```python
from build123d import *

# Parameters (mm, degrees)
SKETCH1_W           = 152.4
SKETCH1_H           = 457.2
SKETCH1_R           = 1.905
BOSS_EXTRUDE1_DEPTH = 4.7625
CUT_EXTRUDE1_REACH  = 411.779
SKETCH3_R           = 1.905
CUT_EXTRUDE4_REACH  = 411.779
SKETCH6_W           = 120.6373
SKETCH6_H           = 44.403792
SKETCH6_H_2         = 44.496208
SKETCH7_R           = 1.905
CUT_EXTRUDE5_DEPTH  = 410.778918528


with BuildPart() as part:
    # Sketch1 → Boss-Extrude1 (new body)
    with BuildSketch(Plane.XY):
        with Locations((-118.546343616, 131.913442623)):
            Rectangle(SKETCH1_W, SKETCH1_H)
        with Locations(Location((-61.396343616, 346.238642623, 0), (0, 0, 180))):
            Circle(SKETCH1_R, mode=Mode.SUBTRACT)
        with Locations(Location((-180.471543616, 346.238642623, 0), (0, 0, 180))):
            Circle(SKETCH1_R, mode=Mode.SUBTRACT)
        with Locations(Location((-180.471543616, -82.411757377, 0), (0, 0, 180))):
            Circle(SKETCH1_R, mode=Mode.SUBTRACT)
        with Locations(Location((-61.396343616, -82.411757377, 0), (0, 0, 180))):
            Circle(SKETCH1_R, mode=Mode.SUBTRACT)
    extrude(amount=BOSS_EXTRUDE1_DEPTH)

    # Sketch3 → Cut-Extrude1 (cut, up to next)
    with BuildSketch(Plane.XY.offset(4.7625), mode=Mode.PRIVATE) as cut_extrude1_sk1:
        with Locations((-156.633643616, 182.654534623)):
            Circle(SKETCH3_R)
    cut_extrude1_tool1 = extrude(cut_extrude1_sk1.sketch, amount=-CUT_EXTRUDE1_REACH, mode=Mode.PRIVATE) & part.part
    # Sketch3 → Cut-Extrude1 (cut, up to next)
    with BuildSketch(Plane.XY.offset(4.7625), mode=Mode.PRIVATE) as cut_extrude1_sk2:
        with Locations((-80.433643616, 182.654534623)):
            Circle(SKETCH3_R)
    cut_extrude1_tool2 = extrude(cut_extrude1_sk2.sketch, amount=-CUT_EXTRUDE1_REACH, mode=Mode.PRIVATE) & part.part
    # Sketch3 → Cut-Extrude1 (cut, up to next)
    with BuildSketch(Plane.XY.offset(4.7625), mode=Mode.PRIVATE) as cut_extrude1_sk3:
        with Locations((-156.633643616, 81.054534623)):
            Circle(SKETCH3_R)
    cut_extrude1_tool3 = extrude(cut_extrude1_sk3.sketch, amount=-CUT_EXTRUDE1_REACH, mode=Mode.PRIVATE) & part.part
    # Sketch3 → Cut-Extrude1 (cut, up to next)
    with BuildSketch(Plane.XY.offset(4.7625), mode=Mode.PRIVATE) as cut_extrude1_sk4:
        with Locations((-80.433643616, 81.054534623)):
            Circle(SKETCH3_R)
    cut_extrude1_tool4 = extrude(cut_extrude1_sk4.sketch, amount=-CUT_EXTRUDE1_REACH, mode=Mode.PRIVATE) & part.part
    add(cut_extrude1_tool1.solids().sort_by_distance((-156.633644, 182.654535, 4.7625))[0], mode=Mode.SUBTRACT)
    add(cut_extrude1_tool2.solids().sort_by_distance((-80.433644, 182.654535, 4.7625))[0], mode=Mode.SUBTRACT)
    add(cut_extrude1_tool3.solids().sort_by_distance((-156.633644, 81.054535, 4.7625))[0], mode=Mode.SUBTRACT)
    add(cut_extrude1_tool4.solids().sort_by_distance((-80.433644, 81.054535, 4.7625))[0], mode=Mode.SUBTRACT)

    # Sketch6 → Cut-Extrude4 (cut, up to next)
    with BuildSketch(Plane.XY.offset(4.7625), mode=Mode.PRIVATE) as cut_extrude4_sk1:
        with Locations((-118.539993616, 42.977638623)):
            Rectangle(SKETCH6_W, SKETCH6_H)
    cut_extrude4_tool1 = extrude(cut_extrude4_sk1.sketch, amount=-CUT_EXTRUDE4_REACH, mode=Mode.PRIVATE) & part.part
    # Sketch6 → Cut-Extrude4 (cut, up to next)
    with BuildSketch(Plane.XY.offset(4.7625), mode=Mode.PRIVATE) as cut_extrude4_sk2:
        with Locations((-118.539993616, 220.777638623)):
            Rectangle(SKETCH6_W, SKETCH6_H_2)
    cut_extrude4_tool2 = extrude(cut_extrude4_sk2.sketch, amount=-CUT_EXTRUDE4_REACH, mode=Mode.PRIVATE) & part.part
    add(cut_extrude4_tool1.solids().sort_by_distance((-118.539994, 42.977639, 4.7625))[0], mode=Mode.SUBTRACT)
    add(cut_extrude4_tool2.solids().sort_by_distance((-118.539994, 220.777639, 4.7625))[0], mode=Mode.SUBTRACT)

    # Sketch7 → Cut-Extrude5 (cut, through all)
    with BuildSketch(Plane.XY.offset(4.7625)):
        with Locations((-157.236735827, -7.432198967)):
            Circle(SKETCH7_R)
        with Locations((-156.646343616, -45.899257377)):
            Circle(SKETCH7_R)
        with Locations((-80.446343616, -45.899257377)):
            Circle(SKETCH7_R)
        with Locations((-80.446343616, -7.799257377)):
            Circle(SKETCH7_R)
        with Locations((-79.900784131, 271.600742623)):
            Circle(SKETCH7_R)
        with Locations((-79.900784131, 309.700742623)):
            Circle(SKETCH7_R)
        with Locations((-156.100784131, 309.700742623)):
            Circle(SKETCH7_R)
        with Locations((-156.100784131, 271.600742623)):
            Circle(SKETCH7_R)
    extrude(amount=-CUT_EXTRUDE5_DEPTH, mode=Mode.SUBTRACT)


solid = part.part
```
Verification items for the finished model (mm, model axes). Give positions to 0.01 mm unless a question says otherwise; leave off trailing zeros. Order: outer loops, then holes, each group sorted by start corner. A loop starts at its lowest first (then second) coordinate and runs counter-clockwise, first axis right, second up. Notation, with made-up numbers: (-31.75, 47) -> (8.25, 47) arc R28 ccw to (8.25, 81) -> close; hole circle Ø2 at (16.25, 13.25). An arc over 180 degrees is marked (long way). One line per item, written item: value.
(1) Sectioned sample at B-B on z = 1.7. Count the separate pieces of the cut face and the enclosed holes in it, then the cut area to 3 significant figures.
Final values:
separate pieces: 1
enclosed holes: 18
area: 58,800 mm^2
(2) Scan lines: line 1 along Y through (x, z) = (-90, 3.95); line 2 along X through (y, z) = (50.5, 1.5); line 3 along X through (y, z) = (-45, 0.7). Record each from-to range of solid material in increasing order. Write a range as [from, to].
Final values:
line 1: [-96.69, 20.78], [65.18, 198.53], [243.03, 360.51]
line 2: [-194.75, -178.86], [-58.22, -42.35]
line 3: [-194.75, -158.33], [-154.97, -82.13], [-78.77, -42.35]
(3) Sectioned sample at A-A on x = -88.5. Record the cut outline in (y, z), then the cut area to 3 significant figures.
Final values:
outline: (-96.69, 0) -> (20.78, 0) -> (20.78, 4.76) -> (-96.69, 4.76) -> close; (65.18, 0) -> (198.53, 0) -> (198.53, 4.76) -> (65.18, 4.76) -> close; (243.03, 0) -> (360.51, 0) -> (360.51, 4.76) -> (243.03, 4.76) -> close
area: 1,750 mm^2
(4) Gauge pin test, flat end, axial feed: pin 1 (3.5 mm diameter, centred on x = -79.9, y = 309.7, fed in from +Z). Record the tip position at first contact, or that the pin passes through.
Final values:
pin 1: through
